Can you work these out from the drawing? Everything is in mm from the part's minimum corner. Coordinates: 2 decimals unless noted, no trailing zeros. Loops run counter-clockwise (first coordinate to the right, second up) from the corner with the lowest first, then second, coordinate; pieces in that order, holes last. Notation, with made-up numbers: M 1.25,71 L 29.25,71 A6 ccw 29.25,81 Z; hole C -3.75,18 d8. An arc over 180 degrees is marked long. Use CSV: the item, a comma, the result in double quotes. Start each with the question number.
Q1. If we section it at D-D (y = 60): Please give me the cut outline in (x, z) (3 decimals).
Q2. If we mould it in two halves opening along X, with no side actions, what happens to the marked faces 1, 2, 3 and 4? For each: +X half, -X half, draft (parallel to the pull), parting line (faces both ways), or undercut.
Q3. If we section it at A-A (y = 75): Please give me the cut outline in (x, z) (1 decimal), and give its area (3 significant figures).
Q4. If we section it at C-C (z = 7.75): Please give me the cut outline in (x, y) (1 decimal), and give its area (3 significant figures).
Q5. Please list where these lines run through material, in increasing order: probe 1 along Y at (x, z) = (5, 3.5) (1 decimal); probe 2 along Y at (x, z) = (20, 9) (3 decimals); probe 3 along X at (y, z) = (75, 8.5) (1 decimal). Write a range as [from, to].
Q6. For pin 1 Ø6.5 at (x, y) = (35, 5) entering from +Z; pin 2 Ø3 at (x, y) = (10.5, 57) entering from -Z, each with a flat end and sliding along its axis, tell me the tip position at first contact or that it passes through.
Q7. If we section it at B-B (x = 20): Please give me the cut outline in (y, z) (3 decimals), and give its area (3 significant figures).
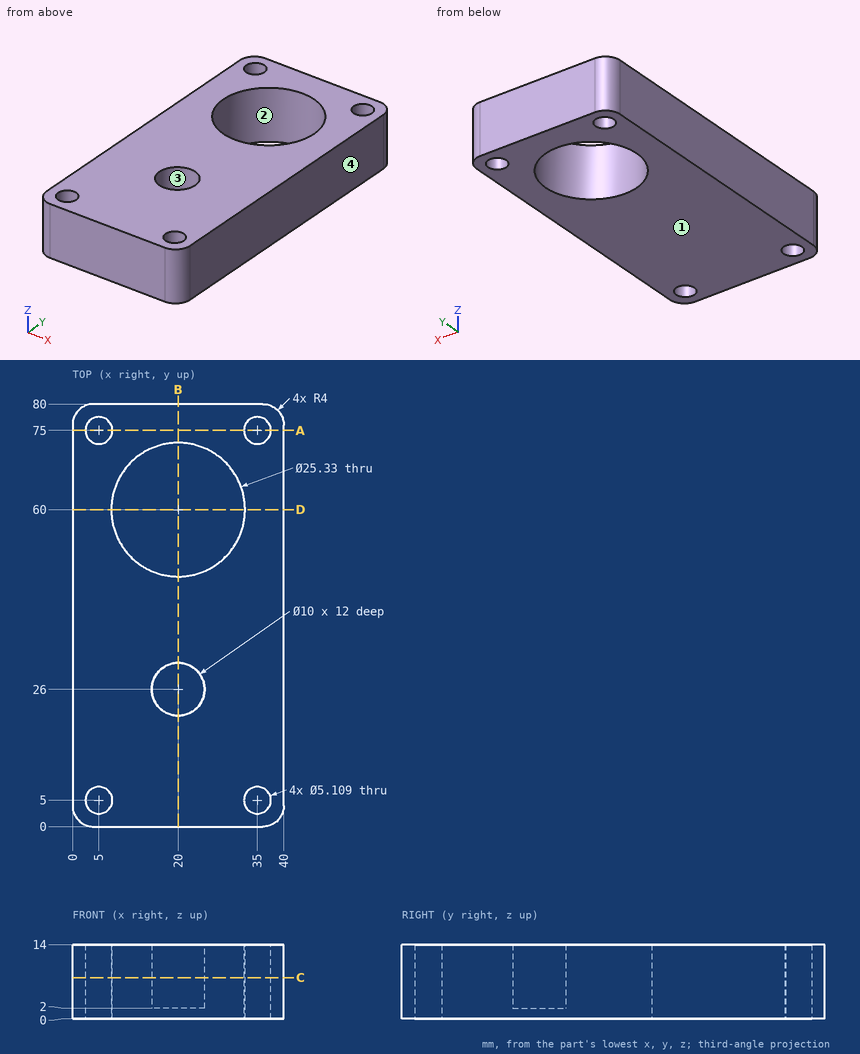
Results below:
1,outline,"M 0,0 L 7.335,0 L 7.335,14 L 0,14 Z; M 32.665,0 L 40,0 L 40,14 L 32.665,14 Z"
2,face 1,"draft"
2,face 2,"undercut"
2,face 3,"undercut"
2,face 4,"+X half"
3,outline,"M 0,0 L 2.4,0 L 2.4,14 L 0,14 Z; M 7.6,0 L 32.4,0 L 32.4,14 L 7.6,14 Z; M 37.6,0 L 40,0 L 40,14 L 37.6,14 Z"
3,area,"417 mm^2"
4,outline,"M 0,4 A4 ccw 4,0 L 36,0 A4 ccw 40,4 L 40,76 A4 ccw 36,80 L 4,80 A4 ccw 0,76 Z; hole C 5,5 d5.1; hole C 5,75 d5.1; hole C 20,60 d25.3; hole C 20,26 d10; hole C 35,5 d5.1; hole C 35,75 d5.1"
4,area,"2,520 mm^2"
5,probe 1,"[0, 2.4], [7.6, 72.4], [77.6, 80]"
5,probe 2,"[0, 21], [31, 47.335], [72.665, 80]"
5,probe 3,"[0, 2.4], [7.6, 32.4], [37.6, 40]"
6,pin 1,"z = 14"
6,pin 2,"through"
7,outline,"M 0,0 L 47.335,0 L 47.335,14 L 31,14 L 31,2 L 21,2 L 21,14 L 0,14 Z; M 72.665,0 L 80,0 L 80,14 L 72.665,14 Z"
7,area,"645 mm^2"
